from build123d import *

# Parameters (mm, degrees)
M10_CLEARANCE_HOLE1_D = 11
CIRPATTERN1_COUNT     = 4


with BuildPart() as part:
    # Sketch5 → Revolve1 (revolve)
    with BuildSketch(Plane(origin=(0, 0, 0), x_dir=(0, 0, -1), z_dir=(1, 0, 0))):
        Polygon((34.85, 6), (95, 6), (95, 0), (0, 0), (0, 26), (22.85, 26), (22.85, 16), (34.85, 16), align=None)
    revolve(axis=Axis((0, 0, 0), (0, 1, 0)))

    # M10 Clearance Hole1 (through all)
    with Locations(Plane(origin=(0, 6, -80), x_dir=(0, 0, 1), z_dir=(0, 1, 0))):
        with Locations((0, 0)):
            m10_clearance_hole1 = Hole(M10_CLEARANCE_HOLE1_D / 2)

    # CirPattern1: M10 Clearance Hole1 ×4 about axis
    cirpattern1_axis = Axis((0, 0, 0), (0, 1, 0))
    for i in range(1, CIRPATTERN1_COUNT):
        add(m10_clearance_hole1.rotate(cirpattern1_axis, i * 360 / CIRPATTERN1_COUNT), mode=Mode.SUBTRACT)


solid = part.part
Source: CAD feature listing. Evaluate the final solid. Frame: model axes, mm. A direction names the side the tool comes from. Give positions to 0.01 mm unless a question says otherwise; leave off trailing zeros. Order: outer loops, then holes, each group sorted by start corner. A loop starts at its lowest first (then second) coordinate and runs counter-clockwise, first axis right, second up. Notation, with made-up numbers: (30.25, 4.25) -> (89.25, 4.25) arc R22 ccw to (89.25, 17.25) -> close; hole circle Ø7 at (21.5, -2.5). An arc over 180 degrees is marked (long way). Use a Markdown table: item, result.
1) Section query A-A, the plane z = 0. Return the cut outline in (x, y), then the cut area to 3 significant figures.
Answer list:
| item | result |
|---|---|
| outline | (-95, 0) -> (-85.5, 0) -> (-85.5, 6) -> (-95, 6) -> close; (-74.5, 0) -> (74.5, 0) -> (74.5, 6) -> (34.85, 6) -> (34.85, 16) -> (22.85, 16) -> (22.85, 26) -> (-22.85, 26) -> (-22.85, 16) -> (-34.85, 16) -> (-34.85, 6) -> (-74.5, 6) -> close; (85.5, 0) -> (95, 0) -> (95, 6) -> (85.5, 6) -> close |
| area | 2,160 mm² |
2) Reachability of faces 1 (the cylindrical face through (-15.443, 20.93, 16.841)), 2 (the cylindrical face through (74.505, 2.958, 0.242)) from +Z, -Z, +X, -X, +Y, -Y: full face, straight path, thin tool, end or side. Return the list, or none.
Answer list:
| item | result |
|---|---|
| face 1 | +Y |
| face 2 | +Y, -Y |
3) Contact query for flat-ended pins moving along their axis: P1, Ø8, axis at y = 16.5, z = -28.5, coming from the -X side; P2, Ø2, axis at x = -15.5, y = 14.5, coming from the -Z side; P3, Ø1, axis at x = -52.5, z = -53, coming from the +Y side; P4, Ø4, axis at x = 56, z = 35.5, coming from the -Y side. Output: stop coordinate, or through.
Answer list:
| item | result |
|---|---|
| P1 | x = -24.75 |
| P2 | z = -31.69 |
| P3 | y = 6 |
| P4 | y = 0 |
4) Section query C-C, the plane z = 80. Return the cut outline in (x, y), then the cut area to 3 significant figures.
Answer list:
| item | result |
|---|---|
| outline | (-51.23, 0) -> (-5.5, 0) -> (-5.5, 6) -> (-51.23, 6) -> close; (5.5, 0) -> (51.23, 0) -> (51.23, 6) -> (5.5, 6) -> close |
| area | 549 mm² |
5) Section query B-B, the plane x = -80. Return the cut outline in (y, z).
Answer list:
| item | result |
|---|---|
| outline | (0, -51.23) -> (6, -51.23) -> (6, -5.5) -> (0, -5.5) -> close; (0, 5.5) -> (6, 5.5) -> (6, 51.23) -> (0, 51.23) -> close |
6) Section query D-D, the plane y = 3.25. Return the cut outline in (x, z), then the cut area to 3 significant figures.
Answer list:
| item | result |
|---|---|
| outline | circle Ø190 at (0, 0); hole circle Ø11 at (-80, 0); hole circle Ø11 at (0, -80); hole circle Ø11 at (0, 80); hole circle Ø11 at (80, 0) |
| area | 28,000 mm² |
7) Mould query, pull axis X, two halves, no side actions, for faces 3 (the cylindrical face through (-0.242, 2.958, 74.505)), 4 (the cylindrical face through (92.74, 2.96, 20.59)), 5 (the flat face through (23, 16, 7)). Classes: +X half, -X half, draft (parallel to the pull), parting line (faces both ways), or undercut.
Answer list:
| item | result |
|---|---|
| face 3 | undercut |
| face 4 | parting line |
| face 5 | draft |
8) Ray query, line 1 along X through (y, z) = (2.85, 80); line 2 along Z through (x, y) = (1, 17.25); line 3 along Y through (x, z) = (-44, -51). Return the intervals inside material, ascending. Write a range as [from, to].
Answer list:
| item | result |
|---|---|
| line 1 | [-51.23, -5.5], [5.5, 51.23] |
| line 2 | [-22.83, 22.83] |
| line 3 | [0, 6] |
